Check sheet for the modelled part. Datum: model origin and axes. Units: mm. Give positions to 0.01 mm unless a question says otherwise; leave off trailing zeros. Order: outer loops, then holes, each group sorted by start corner. A loop starts at its lowest first (then second) coordinate and runs counter-clockwise, first axis right, second up. Notation, with made-up numbers: (-27, 40.25) -> (19, 40.25) arc R26 cw to (19, 79.25) -> close; hole circle Ø7 at (82, 32.25). An arc over 180 degrees is marked (long way). Answer in a Markdown table with one row per item. Add a question column.
(1) Cross-section at C-C (z = 3.25). Record the cut outline in (x, y).
(2) Cross-section at A-A (y = 50.5). Record the cut outline in (x, z), then the cut area to 3 significant figures.
(3) Release check for a two-part mould opening along Y. For faces 1 (the face through (22, 0, 4)), 2 (the face through (0, 27, 4)), 3 (the face through (20.9, 2.8, 4.1)) record: released by +Y, released by -Y, zero draft, split by the parting line, or undercut.
(4) Cross-section at D-D (x = 34.5). Record the cut outline in (y, z).
(5) Thickness scan on L1, parallel to Y at x = 10.5, z = 2.5; L2, parallel to Y at x = 35, z = 5.25; L3, parallel to X at y = 5.5, z = 0.5. Record the ranges inside material, lowest first. Write a range as [from, to].
(6) Go/stop test with a flat-tipped pin: pin 1 (3 mm diameter, centred on x = 22.5, y = 50.5, fed in from -Z). Record where the tip stops, or that it passes through.
(7) Cross-section at B-B (x = 11.5). Record the cut outline in (y, z).
```python
from build123d import *

# Parameters (mm, degrees)
ESQUISSE1_W             = 45
ESQUISSE1_H             = 54.5
BOSS_EXTRU_1_DEPTH      = 8
ESQUISSE2_R             = 2
ENL_V_MAT_EXTRU_1_DEPTH = 8


with BuildPart() as part:
    # Esquisse1 → Boss.-Extru.1 (new body)
    with BuildSketch(Plane.XY):
        with Locations((22.5, 27.25)):
            Rectangle(ESQUISSE1_W, ESQUISSE1_H)
    extrude(amount=BOSS_EXTRU_1_DEPTH)

    # Esquisse2 → Enlèv. mat.-Extru.1 (cut)
    with BuildSketch(Plane.XY.offset(8)):
        with Locations(Location((10.5, 4, 0), (0, 0, 180))):
            Circle(ESQUISSE2_R)
        with Locations((34.5, 4)):
            Circle(ESQUISSE2_R)
        with Locations((22.5, 4)):
            Circle(ESQUISSE2_R)
        with Locations(Location((22.5, 50.5, 0), (0, 0, 180))):
            Circle(ESQUISSE2_R)
        with Locations(Location((34.5, 50.5, 0), (0, 0, 180))):
            Circle(ESQUISSE2_R)
        with Locations((10.5, 50.5)):
            Circle(ESQUISSE2_R)
    extrude(amount=-ENL_V_MAT_EXTRU_1_DEPTH, mode=Mode.SUBTRACT)


solid = part.part
```
Answer below:
| question | item | result |
|---|---|---|
| 1 | outline | (0, 0) -> (45, 0) -> (45, 54.5) -> (0, 54.5) -> close; hole circle Ø4 at (10.5, 4); hole circle Ø4 at (10.5, 50.5); hole circle Ø4 at (22.5, 4); hole circle Ø4 at (22.5, 50.5); hole circle Ø4 at (34.5, 4); hole circle Ø4 at (34.5, 50.5) |
| 2 | outline | (0, 0) -> (8.5, 0) -> (8.5, 8) -> (0, 8) -> close; (12.5, 0) -> (20.5, 0) -> (20.5, 8) -> (12.5, 8) -> close; (24.5, 0) -> (32.5, 0) -> (32.5, 8) -> (24.5, 8) -> close; (36.5, 0) -> (45, 0) -> (45, 8) -> (36.5, 8) -> close |
| 2 | area | 264 mm² |
| 3 | face 1 | released by -Y |
| 3 | face 2 | zero draft |
| 3 | face 3 | undercut |
| 4 | outline | (0, 0) -> (2, 0) -> (2, 8) -> (0, 8) -> close; (6, 0) -> (48.5, 0) -> (48.5, 8) -> (6, 8) -> close; (52.5, 0) -> (54.5, 0) -> (54.5, 8) -> (52.5, 8) -> close |
| 5 | L1 | y = [0, 2], [6, 48.5], [52.5, 54.5] |
| 5 | L2 | y = [0, 2.06], [5.94, 48.56], [52.44, 54.5] |
| 5 | L3 | x = [0, 9.18], [11.82, 21.18], [23.82, 33.18], [35.82, 45] |
| 6 | pin 1 | passes through |
| 7 | outline | (0, 0) -> (2.27, 0) -> (2.27, 8) -> (0, 8) -> close; (5.73, 0) -> (48.77, 0) -> (48.77, 8) -> (5.73, 8) -> close; (52.23, 0) -> (54.5, 0) -> (54.5, 8) -> (52.23, 8) -> close |
